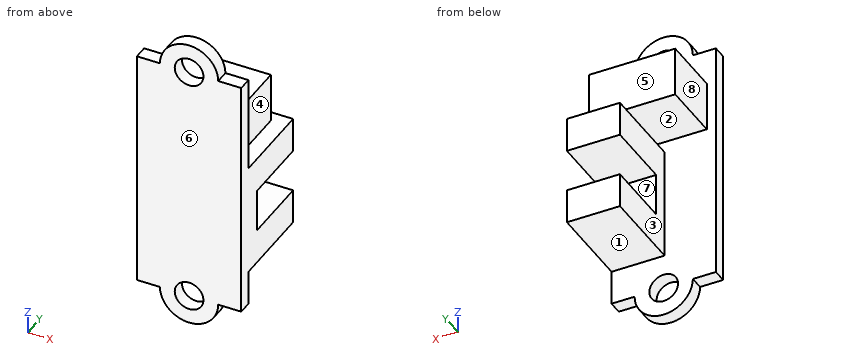
Autodesk Inventor part; units mm, degrees
ref_plane "YZ Plane" through (0, 0, 0) normal (1, 0, 0) x (0, 1, 0)
ref_plane "XZ Plane" through (0, 0, 0) normal (0, 1, 0) x (-1, 0, 0)
ref_plane "XY Plane" through (0, 0, 0) normal (0, 0, 1) x (1, 0, 0)
sketch "草圖1" plane through (0, 0, 0) normal (0, 1, 0) x (-1, 0, 0)
  line L0 (6, 14) -> (6, -14)
  line L1 (-6, -14) -> (-6, 14)
  line L2 (-6, 14) -> (6, -14) construction
  line L3 (6, 14) -> (-6, -14) construction
  circle A0 centre (0, 14) radius 1.65
  circle A1 centre (0, -14) radius 1.65
  arc A2 (-3.35, -14) -> (3.35, -14) centre (0, -14) ccw
  arc A3 (3.35, 14) -> (-3.35, 14) centre (0, 14) ccw
  line L4 (-6, 14) -> (-3.35, 14)
  line L5 (1.65, 14) -> (6, 14)
  line L6 (6, -14) -> (3.35, -14)
  line L7 (-3.35, -14) -> (-6, -14)
  point P0 (0, 0)
  dimension "d2" = 3.3
  dimension "d0" = 12
  dimension "d1" = 28
  dimension "d3" = 3.3
  dimension "d4" = 6.7
  dimension "d5" = 6.7
extrude "擠出1" add sketch "草圖1" along normal blind 1.58
sketch "草圖2" plane through (6, 0, 14) normal (1, 0, 0) x (0, 0, -1)
  line L0 (0, 0) -> (28, 0)
  line L1 (28, 0) -> (28, 1.58)
  line L2 (0, 1.58) -> (28, 1.58)
  line L3 (0, 0) -> (0, 1.58)
  line L4 (11.06, 1.58) -> (11.06, 11.38)
  line L5 (11.06, 11.38) -> (15.06, 11.38)
  line L6 (15.06, 11.38) -> (15.06, 3.42)
  line L7 (15.06, 3.42) -> (20, 3.42)
  line L8 (20, 3.42) -> (20, 11.38)
  line L9 (20, 11.38) -> (24, 11.38)
  line L10 (24, 11.38) -> (24, 1.58)
  point P0 (14, 0)
  dimension "d8" = 12.94
  dimension "d9" = 4
  dimension "d10" = 4
  dimension "d11" = 4
  dimension "d12" = 7.96
  dimension "d13" = 9.8
extrude "擠出2" add sketch "草圖2" against normal blind 6.1 contours L4 L5 L6 L7 L8 L9 L10 L2
sketch "草圖3" plane through (0, 1.58, 0) normal (0, 1, 0) x (1, 0, 0)
  line L0 (4.95, -9.93) -> (-4.95, -9.93)
  line L1 (-4.95, -9.93) -> (-4.95, -4.21)
  line L2 (-4.95, -4.21) -> (4.95, -4.21)
  line L3 (4.95, -4.21) -> (4.95, -9.93)
  line L4 (4.95, -9.93) -> (-4.95, -4.21) construction
  line L5 (-4.95, -9.93) -> (4.95, -4.21) construction
  line L6 (6, -2.94) -> (-0.1, -2.94)
  line L7 (0, 0) -> (0, -12.3322) construction
  point P0 (0, -7.07)
  dimension "d16" = 1.27
  dimension "d17" = 5.72
  dimension "d18" = 9.9
extrude "擠出3" add sketch "草圖3" along normal blind 6.92
properties part number "optic endstop module"
Input: part model. Units: mm. Frame: model coordinates. Face numbers are marked on the shaded views. A direction names the side the tool comes from. Round coordinates to 2 decimals unless told otherwise and drop trailing zeros. Order: outer loops, then holes, each group sorted by start corner. A loop starts at its lowest first (then second) coordinate and runs counter-clockwise, first axis right, second up. Notation, with made-up numbers: (30.25, 86) - (44.25, 86) arc R22 cw to (44.25, 120) - close; hole circle Ø5 at (26.5, 36.5). An arc over 180 degrees is marked (long way). One line per question, with ' | ' between items. Start each with the question number.
1) Ray query, probe 1 along Z at (x, y) = (0, 1.15); probe 2 along Z at (x, y) = (0, 7.25); probe 3 along Z at (x, y) = (3.25, 3). Return the intervals inside material, ascending.
2) Cut plane A-A, the plane y = 3. Return the cut outline in (x, z).
3) Cut plane B-B, the plane x = -4.5. Return the cut outline in (y, z).
4) Pull-direction query (Z, two-part tool) for the marked faces 1, 2 and 3; classes: +Z half, -Z half, draft (parallel to the pull), parting line (faces both ways), or undercut.
5) Cut plane C-C, the plane z = 15. Return the cut outline in (x, y).
6) Contact query for flat-ended pins moving along their axis: P1, Ø1.7, axis at y = 3.5, z = 7.5, coming from the +X side; P2, Ø0.8, axis at x = -5, y = 1, coming from the +Z side; P3, Ø5, axis at x = 2.5, y = 6, coming from the -Z side; P4, Ø3, axis at y = 8, z = -3, coming from the -X side. Output: stop coordinate, or through.
7) Set-up query: the marked faces 4, 5, 6, 7 and 8. Return all of +Z, -Z, +X, -X, +Y, -Y with unobstructed straight access to the full face (end or side cutting, diameter ignored); none if empty.
8) Cut plane D-D, the plane z = -6.5. Return the cut outline in (x, y), then the cut area to 3 significant figures.
Worked out:
1) probe 1: z = -17.35 to -15.65, -12.35 to 12.35, 15.65 to 17.35 | probe 2: z = -10 to -6, -1.06 to 2.94, 4.21 to 9.93 | probe 3: z = -10 to 2.94, 4.21 to 9.93
2) outline: (-4.95, 4.21) - (4.95, 4.21) - (4.95, 9.93) - (-4.95, 9.93) - close; (-0.1, -10) - (6, -10) - (6, 2.94) - (-0.1, 2.94) - close
3) outline: (0, -14) - (1.58, -14) - (1.58, 4.21) - (8.5, 4.21) - (8.5, 9.93) - (1.58, 9.93) - (1.58, 14) - (0, 14) - close
4) face 1: -Z half | face 2: undercut | face 3: draft
5) outline: (-3.2, 0) - (-1.31, 0) - (-1.31, 1.58) - (-3.2, 1.58) - close; (1.31, 0) - (3.2, 0) - (3.2, 1.58) - (1.31, 1.58) - close
6) P1: stops at x = 4.95 | P2: stops at z = 14 | P3: stops at z = -10 | P4: passes through
7) face 4: +Z, +X, +Y | face 5: +Z, +X, -X, +Y | face 6: +Z, -Z, +X, -X, -Y | face 7: +X, -X, +Y | face 8: +Z, -Z, -X, +Y
8) outline: (-6, 0) - (6, 0) - (6, 11.38) - (-0.1, 11.38) - (-0.1, 1.58) - (-6, 1.58) - close | area: 78.7 mm^2
